Input: dimensioned drawing with shaded views. Units: mm. Origin: part minimum x, y, z. Round coordinates to 2 decimals unless told otherwise and drop trailing zeros. Loops run counter-clockwise (first coordinate to the right, second up) from the corner with the lowest first, then second, coordinate; pieces in that order, holes last. Notation, with made-up numbers: (26, 57.5) - (60, 57.5) arc R12 cw to (60, 61.5) - close; hole circle Ø5 at (0, 82.5). An arc over 180 degrees is marked (long way). One line per question, with ' | ' between items. Start each with the question number.
1. Ray query, line 1 (Z direction, x = 45, y = 3.4); line 2 (X direction, y = 7, z = 61); line 3 (X direction, y = 1.5, z = 44). Return the intervals inside material, ascending.
2. Cut plane D-D (x = 12). Return loops of the section in (y, z).
3. Pin query (flat end, axial travel): pin 1 (5.5 mm diameter, centred on x = 65, z = 60, fed in from -Y); pin 2 (4 mm diameter, centred on x = 23.5, z = 47, fed in from +Y); pin 3 (2.5 mm diameter, centred on y = 8, z = 7.5, fed in from -X); pin 4 (1.5 mm diameter, centred on x = 76.5, y = 6.5, fed in from -Z). Return the tip coordinate at first contact, or that it passes through.
4. Cut plane A-A (y = 7). Return loops of the section in (x, z), then the cut area to 3 significant figures.
5. Cut plane C-C (x = 45). Return loops of the section in (y, z), then the cut area to 3 significant figures.
6. Mould query, pull axis Z, two halves, no side actions, for the marked faces 1 and 2. Classes: pulls with the +Z half, pulls with the -Z half, needs draft (parallel to the pull), parting line crosses it, or undercut.
7. Cut plane B-B (z = 60). Return loops of the section in (x, y), then the cut area to 3 significant figures.
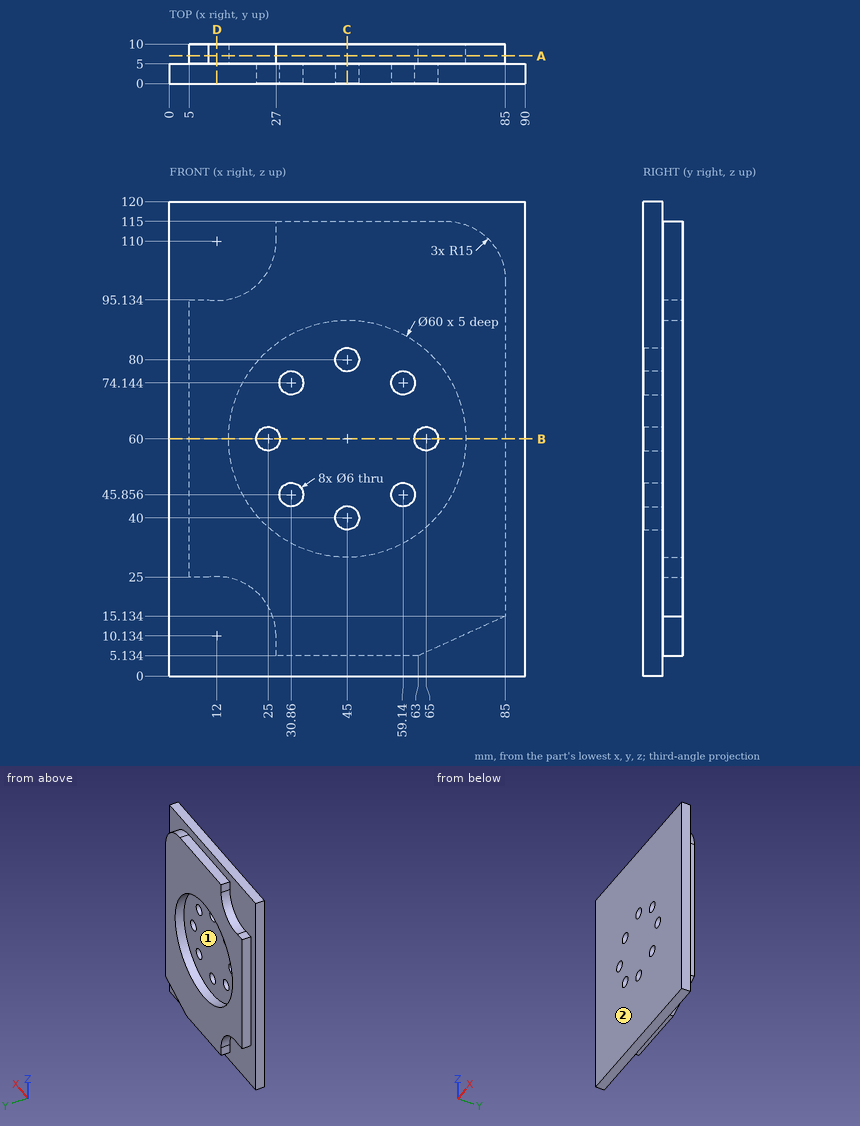
Answers follow:
1) line 1: z = 0 to 37, 43 to 77, 83 to 120 | line 2: x = 5 to 15.02, 74.98 to 85 | line 3: x = 0 to 28.5, 33.22 to 56.78, 61.5 to 90
2) outline: (0, 0) - (5, 0) - (5, 25.13) - (10, 25.13) - (10, 95) - (5, 95) - (5, 120) - (0, 120) - close
3) pin 1: passes through | pin 2: stops at y = 5 | pin 3: stops at x = 27 | pin 4: stops at z = 10.93
4) outline: (5, 25) - (10, 25) arc R15 cw to (27, 10.13) - (27, 5.13) - (63, 5.13) - (85, 15.13) - (85, 100) arc R15 ccw to (70, 115) - (27, 115) - (27, 110) arc R15 cw to (10, 95.13) - (5, 95.13) - close; hole circle Ø60 at (45, 60) | area: 5,020 mm2
5) outline: (0, 0) - (5, 0) - (5, 5.13) - (10, 5.13) - (10, 30) - (5, 30) - (5, 37) - (0, 37) - close; (0, 43) - (5, 43) - (5, 77) - (0, 77) - close; (0, 83) - (5, 83) - (5, 90) - (10, 90) - (10, 115) - (5, 115) - (5, 120) - (0, 120) - close | area: 789 mm2
6) face 1: undercut | face 2: needs draft
7) outline: (0, 0) - (22, 0) - (22, 5) - (15, 5) - (15, 10) - (5, 10) - (5, 5) - (0, 5) - close; (28, 0) - (62, 0) - (62, 5) - (28, 5) - close; (68, 0) - (90, 0) - (90, 5) - (85, 5) - (85, 10) - (75, 10) - (75, 5) - (68, 5) - close | area: 490 mm2
